from build123d import *

# Parameters (mm, degrees)
BOSS_EXTRUDE1_DEPTH      = 9.525
F_0_257_DIAMETER_HOLE1_D = 6.5278
F_1_4_20_TAPPED_HOLE1_D  = 5.1054


with BuildPart() as part:
    # Sketch2 → Boss-Extrude1 (new body)
    with BuildSketch(Plane.XY):
        with BuildLine():
            Line((46.759190155, 52.701629037), (6.061214767, -0.715064976))
            ThreePointArc((6.061214767, -0.715064976), (0, -3.717048568), (-6.061214767, -0.715064976))
            Line((-6.061214767, -0.715064976), (-46.759190155, 52.701629037))
            ThreePointArc((-46.759190155, 52.701629037), (-48.545369458, 54.175208138), (-50.8, 54.702951432))
            Line((-50.8, 54.702951432), (-63.5, 54.702951432))
            Line((-63.5, 54.702951432), (-63.5, 72.482951432))
            Line((-63.5, 72.482951432), (63.5, 72.482951432))
            Line((63.5, 72.482951432), (63.5, 54.702951432))
            Line((63.5, 54.702951432), (50.8, 54.702951432))
            ThreePointArc((50.8, 54.702951432), (48.545369458, 54.175208138), (46.759190155, 52.701629037))
        make_face()
    extrude(amount=BOSS_EXTRUDE1_DEPTH)

    # F (0.257) Diameter Hole1 (through all)
    with Locations(Plane.XY.offset(9.525)):
        with Locations((0, 15.332951432), (-38.1, 53.432951432), (38.1, 53.432951432)):
            Hole(F_0_257_DIAMETER_HOLE1_D / 2)

    # 1/4-20 Tapped Hole1 (through all)
    with Locations(Plane(origin=(0, 72.482951432, 0), x_dir=(1, 0, 0), z_dir=(0, 1, 0))):
        with Locations((-57.15, -4.7625), (57.15, -4.7625)):
            Hole(F_1_4_20_TAPPED_HOLE1_D / 2)


solid = part.part
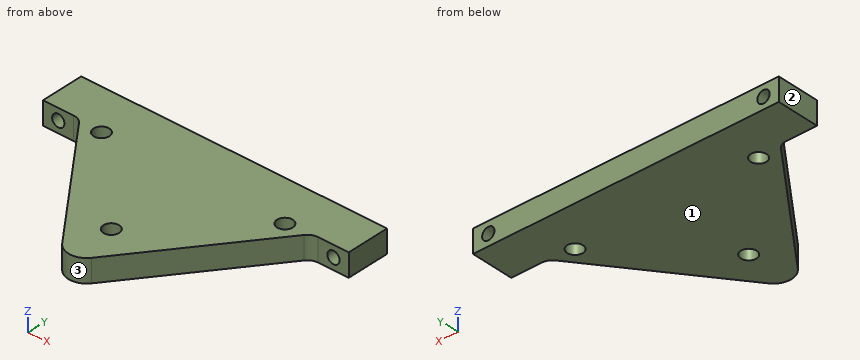
Check sheet for the modelled part. Datum: model origin and axes. Units: mm. Face numbers are marked on the shaded views. Round coordinates to 2 decimals unless told otherwise and drop trailing zeros. Order: outer loops, then holes, each group sorted by start corner. A loop starts at its lowest first (then second) coordinate and runs counter-clockwise, first axis right, second up.
(1) Draft check along X on the marked faces 1, 2 and 3. Enter one of: pulls with the +X half, pulls with the -X half, needs draft (parallel to the pull), parting line crosses it, or undercut.
(2) Go/stop test with flat-tipped pins: P1, Ø4.5, axis at x = 57.15, z = 4.76, coming from the +Y side; P2, Ø4, axis at x = -2.5, z = 4.5, coming from the -Y side. Record where each tip stops, or that it passes through.
(3) Scan lines: probe 1 along Z at (x, y) = (57, 62) (3 decimals); probe 2 along Y at (x, z) = (-38.1, 4.5); probe 3 along Y at (x, z) = (-54, 8.75). Record each from-to range of solid material in increasing order.
(4) Cross-section at D-D, the plane y = 4. Enter the section's corners in (x, z) (3 decimals), and give its area (3 significant figures).
(5) Cross-section at B-B, the plane x = 0. Enter the section's corners in (y, z) (3 decimals), and give its area (3 significant figures).
(6) Cross-section at C-C, the plane y = 65. State how many separate pieces and enclosed holes the cut face has, and give its area (3 significant figures).
(7) Cross-section at A-A, the plane x = 57.15. Enter the section's corners in (y, z) (3 decimals), and give its area (3 significant figures).
Check sheet entries:
1. face 1: needs draft
1. face 2: pulls with the -X half
1. face 3: parting line crosses it
2. P1: passes through
2. P2: stops at y = -3.7
3. probe 1: z = 0 to 2.214, 7.311 to 9.525
3. probe 2: y = 41.34 to 50.17, 56.7 to 72.48
3. probe 3: y = 54.7 to 72.48
4. outline: (-9.654, 0) - (9.654, 0) - (9.654, 9.525) - (-9.654, 9.525) - close
4. area: 184 mm2
5. outline: (-3.717, 0) - (12.069, 0) - (12.069, 9.525) - (-3.717, 9.525) - close; (18.597, 0) - (72.483, 0) - (72.483, 9.525) - (18.597, 9.525) - close
5. area: 664 mm2
6. separate pieces: 1
6. enclosed holes: 2
6. area: 1,170 mm2
7. outline: (54.703, 0) - (72.483, 0) - (72.483, 2.21) - (54.703, 2.21) - close; (54.703, 7.315) - (72.483, 7.315) - (72.483, 9.525) - (54.703, 9.525) - close
7. area: 78.6 mm2
